Part model, mm, in its own coordinate system. Give positions to 0.01 mm unless a question says otherwise; leave off trailing zeros. Order: outer loops, then holes, each group sorted by start corner. A loop starts at its lowest first (then second) coordinate and runs counter-clockwise, first axis right, second up. Notation, with made-up numbers: (11, -4) - (70, -4) arc R16 cw to (70, 18) - close; hole circle Ø9 at (45, 74). An arc over 180 degrees is marked (long way). One line per item, written item: value.
Autodesk Inventor part; units mm, degrees
ref_plane "YZ Plane" through (0, 0, 0) normal (1, 0, 0) x (0, 1, 0)
ref_plane "XZ Plane" through (0, 0, 0) normal (0, 1, 0) x (-1, 0, 0)
ref_plane "XY Plane" through (0, 0, 0) normal (0, 0, 1) x (1, 0, 0)
sketch "Sketch1" plane through (0, 0, 0) normal (0, 0, 1) x (1, 0, 0)
  line L0 (4.5995, 3.2228) -> (80.3423, 3.2228)
  line L1 (80.3423, 3.2228) -> (80.3423, 65.9862)
  line L2 (80.3423, 65.9862) -> (4.5995, 65.9862)
  line L3 (4.5995, 65.9862) -> (4.5995, 3.2228)
  point P0 (0, 0)
  dimension "d0" = 75.7428
  dimension "d1" = 62.7634
extrude "Extrusion1" add sketch "Sketch1" along normal blind 0.7937
sketch "Sketch4" plane through (0, 0, 0.7937) normal (0, 0, 1) x (1, 0, 0)
  line L0 (4.5995, 3.2228) -> (4.5995, 65.9862)
  line L1 (4.5995, 65.9862) -> (80.3423, 65.9862)
  line L2 (4.5995, 52.067) -> (14.2094, 52.067)
  line L3 (14.2094, 52.067) -> (14.2094, 26.667)
  line L4 (14.2094, 26.667) -> (4.5995, 26.667)
  line L5 (4.5995, 26.667) -> (4.5995, 52.067)
  point P0 (0, 0)
  dimension "d18" = 13.9192
  dimension "d19" = 25.4
extrude "Extrusion4" cut sketch "Sketch4" against normal through all
sketch "Sketch5" plane through (0, 0, 0.7937) normal (0, 0, 1) x (1, 0, 0)
  line L0 (4.5995, 65.9862) -> (80.3423, 65.9862)
  line L1 (4.5995, 52.067) -> (4.5995, 65.9862)
  circle A0 centre (19.0208, 61.2935) radius 3.175
  circle A1 centre (19.0208, 48.7936) radius 3.175
  circle A2 centre (19.0208, 36.0437) radius 3.175
  circle A3 centre (19.0208, 23.5438) radius 3.175
  point P0 (0, 0)
  dimension "d20" = 6.35
  dimension "d21" = 14.4213
  dimension "d28" = 12.4999
  dimension "d29" = 12.7499
  dimension "d30" = 12.4999
  dimension "d31" = 4.6927
extrude "Extrusion5" cut sketch "Sketch5" against normal through all
equation "\"d30\" = d28"
properties part number "lcd_standoff"
1) Slice it at B-B on z = 0.25. Count the separate pieces of the cut face and the enclosed holes in it, then the cut area to 3 significant figures.
Answer:
separate pieces: 1
enclosed holes: 4
area: 4,380 mm2
2) Drop a flat-ended pin along its axis: P1, Ø7.5, axis at x = 19.02, y = 23.54, coming from the +Z side. Give the stop position or say it passes through.
Answer:
P1: stops at z = 0.79
3) Slice it at C-C on y = 34. Write the cut outline in (x, z).
Answer:
outline: (14.21, 0) - (16.59, 0) - (16.59, 0.79) - (14.21, 0.79) - close; (21.45, 0) - (80.34, 0) - (80.34, 0.79) - (21.45, 0.79) - close
4) Two-plate mould, pull along Y, no slides. Class faces 1 (the face through (42, 35, 0.794)), 2 (the face through (18.3, 45.7, 0.4)): pulls with the +Y half, pulls with the -Y half, needs draft (parallel to the pull), parting line crosses it, or undercut.
Answer:
face 1: needs draft
face 2: undercut
5) Wall check: line 1 along Y through (x, z) = (19, 0.4); line 2 along Y through (x, z) = (14, 0.6); line 3 along X through (y, z) = (47.5, 0.5). Give the ranges that are in metal, low to high. Write a range as [from, to].
Answer:
line 1: y = [3.22, 20.37], [26.72, 32.87], [39.22, 45.62], [51.97, 58.12], [64.47, 65.99]
line 2: y = [3.22, 26.67], [52.07, 65.99]
line 3: x = [14.21, 16.12], [21.92, 80.34]
6) Slice it at A-A on y = 59. Write the cut outline in (x, z), then the cut area to 3 significant figures.
Answer:
outline: (4.6, 0) - (16.83, 0) - (16.83, 0.79) - (4.6, 0.79) - close; (21.22, 0) - (80.34, 0) - (80.34, 0.79) - (21.22, 0.79) - close
area: 56.6 mm2
